Design review of the part built by this model. Coordinates are the model's own, in mm. A direction names the side the tool comes from. Coordinates: 2 decimals unless noted, no trailing zeros. Write each loop counter-clockwise with the first axis right and the second up, starting at its lowest first coordinate (ties: lowest second). Pieces come first, ordered by that corner, then holes. Notation, with made-up numbers: M 14.25,81.25 L 43.25,81.25 A15 cw 43.25,99.25 Z; hole C 41,15 d7. An arc over 180 degrees is marked long. Return JSON: item names as keys, results as strings. Group by question number.
Autodesk Inventor part; units mm, degrees
ref_plane "YZ Plane" through (0, 0, 0) normal (1, 0, 0) x (0, 1, 0)
ref_plane "XZ Plane" through (0, 0, 0) normal (0, 1, 0) x (-1, 0, 0)
ref_plane "XY Plane" through (0, 0, 0) normal (0, 0, 1) x (1, 0, 0)
ref_plane "작업 평면4" through (0, 0, 0) normal (0, 0, 1) x (1, 0, 0)
sketch "스케치5" plane through (0, 0, 0) normal (0, 0, 1) x (1, 0, 0)
  line L0 (-9.2237, 8.5) -> (-9.2237, -8.5)
  line L1 (-9.2237, -8.5) -> (-15.7763, -8.5)
  line L2 (-15.7763, -8.5) -> (-15.7763, -13)
  line L3 (-15.7763, -13) -> (15.7763, -13)
  line L4 (15.7763, -13) -> (15.7763, -8.5)
  line L5 (15.7763, -8.5) -> (5.2737, -8.5)
  line L6 (5.2737, -8.5) -> (5.2737, 8.5)
  line L7 (5.2737, 8.5) -> (15.7763, 8.5)
  line L8 (15.7763, 8.5) -> (15.7763, 13)
  line L9 (15.7763, 13) -> (-15.7763, 13)
  line L10 (-15.7763, 13) -> (-15.7763, 8.5)
  line L11 (-15.7763, 8.5) -> (-9.2237, 8.5)
  circle A0 centre (2.7487, 0.5) radius 1.6
  line L12 (15.7763, 13) -> (-15.7763, 13)
  line L13 (-15.7763, 13) -> (-15.7763, 8.5)
  line L14 (-15.7763, 8.5) -> (15.7763, 8.5)
  line L15 (15.7763, 8.5) -> (15.7763, 13)
  line L16 (5.2737, 8.5) -> (-9.2237, 8.5)
  line L17 (-9.2237, 8.5) -> (-9.2237, -8.5)
  line L18 (-9.2237, -8.5) -> (5.2737, -8.5)
  line L19 (5.2737, -8.5) -> (5.2737, 8.5)
  line L20 (15.7763, -8.5) -> (-15.7763, -8.5)
  line L21 (-15.7763, -8.5) -> (-15.7763, -13)
  line L22 (-15.7763, -13) -> (15.7763, -13)
  line L23 (15.7763, -13) -> (15.7763, -8.5)
  point P0 (0, 0)
extrude "돌출1" add sketch "스케치5" against normal blind 10
sketch "스케치6" plane through (-15.7763, 13, 0) normal (0, 1, 0) x (1, 0, 0)
  arc A0 (2, 10) -> (0, 8) centre (2, 8) ccw
  line L0 (0, 8) -> (0, 0)
  line L1 (31.5525, 0) -> (0, 0)
  line L2 (31.5525, 10) -> (31.5525, 0)
  line L3 (31.5525, 10) -> (2, 10)
  circle A1 centre (3.025, 7.2) radius 1.35
  circle A2 centre (25.025, 7.2) radius 1.35
  circle A3 centre (25.025, 7.2) radius 1.35
  circle A4 centre (3.025, 7.2) radius 1.35
  point P0 (15.7763, 0)
extrude "돌출2" cut sketch "스케치6" against normal through all contours A1 | A2
fillet "모깎기1" radius 2 2 edges at (-15.7763, 10.75, -10) (-15.7763, -10.75, -10)
properties part number "front ankle connection_right" material "PMMA 플라스틱"
Item 1: Add section D-D (x = 14.5). Write out the cut boundary in (y, z), plus the area to 3 significant figures.
Item 2: Machinability: for faces 1 (the flat face through (5.274, 0, -5)), 2 (the flat face through (-13, 8.5, -5)), 3 (the flat face through (-15.776, -11, -4)), which of the approach directions +Z, -Z, +X, -X, +Y, -Y give a long, thin tool a straight path to every point of the face, cutting with its end or side? Answer none if there is none.
Item 3: For line 1 (X direction, y = -9.85, z = -7.2); line 2 (Y direction, x = -10.5, z = -6.25); line 3 (X direction, y = 11.25, z = -7.75), list the stretches that pass through material, from the lowest coordinate up.
Item 4: The part is to be moulded in two halves that separate along Z. For faces 4 (the cylindrical face through (-13.823, 10.782, -6.379)), 5 (the flat face through (-15.776, 11, -4)), 6 (the flat face through (-2, 0, -10)), 7 (the cylindrical face through (-13.823, -10.718, -6.379)), say which applies: pulls with the +Z half, pulls with the -Z half, needs draft (parallel to the pull), parting line crosses it, or undercut.
Item 5: Add section B-B (z = -2.5). Write out the cut boundary in (x, y), plus the area to 3 significant figures.
Item 6: Add section A-A (z = -7.2). Count the separate pieces of the cut face and the enclosed holes in it, plus the area to 3 significant figures.
Item 7: For pin 1 (12 mm diameter, centred on x = 6, y = -3, fed in from -Z); pin 2 (2 mm diameter, centred on y = 4.5, z = -6.5, fed in from +X); pin 3 (3 mm diameter, centred on y = 2, z = -7, fed in from -X), all flat-tipped, find the tip position at first contact; note any pin that passes through.
Item 8: Add section C-C (y = 0.5). Write out the cut boundary in (x, z).
Geometry check:
{
 "1": {"outline": "M -13,-10 L -8.5,-10 L -8.5,0 L -13,0 Z; M 8.5,-10 L 13,-10 L 13,0 L 8.5,0 Z", "area": "90.0 mm^2"},
 "2": {"face 1": "+Z, -Z, +X", "face 2": "+Z, -Z, -X", "face 3": "+Z, -Z, -X, +Y, -Y"},
 "3": {"line 1": "-15.78 to -14.1, -11.4 to 7.9, 10.6 to 15.78", "line 2": "-13 to -8.5, 8.5 to 13", "line 3": "-15.78 to -13.98, -11.52 to 8.02, 10.48 to 15.78"},
 "4": {"face 4": "undercut", "face 5": "needs draft", "face 6": "pulls with the -Z half", "face 7": "undercut"},
 "5": {"outline": "M -15.78,-13 L 15.78,-13 L 15.78,-8.5 L 5.27,-8.5 L 5.27,8.5 L 15.78,8.5 L 15.78,13 L -15.78,13 L -15.78,8.5 L -9.22,8.5 L -9.22,-8.5 L -15.78,-8.5 Z; hole C 2.75,0.5 d3.2", "area": "522 mm^2"},
 "6": {"separate pieces": "5", "enclosed holes": "1", "area": "474 mm^2"},
 "7": {"pin 1": "z = -10", "pin 2": "x = 5.27", "pin 3": "x = -9.22"},
 "8": {"outline": "M -9.22,-10 L 1.15,-10 L 1.15,0 L -9.22,0 Z; M 4.35,-10 L 5.27,-10 L 5.27,0 L 4.35,0 Z"}
}
